The listing builds one solid part. Answer for the finished solid, in the listing's coordinates (mm). Face numbers are marked on the shaded views. A direction names the side the tool comes from. Coordinates: 2 decimals unless noted, no trailing zeros. Write each loop counter-clockwise with the first axis right and the second up, starting at its lowest first coordinate (ties: lowest second). Pieces come first, ordered by that corner, then holes.
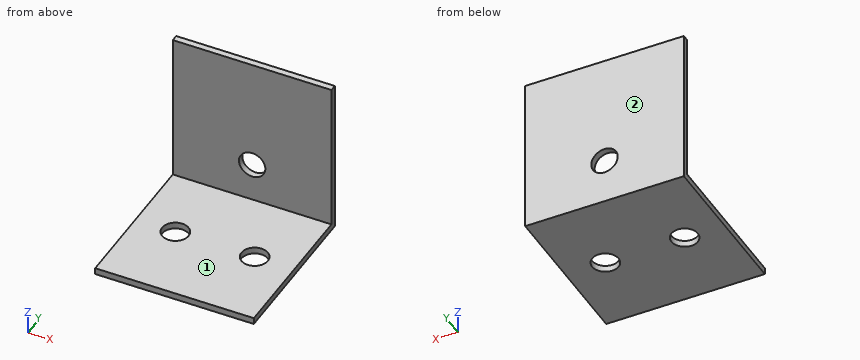
from build123d import *

# Parameters (mm, degrees)
F1_DEPTH = 38.1
F3_D     = 6.35
F5_D     = 6.35


with BuildPart() as f1:
    # F0 (on Right) → F1 (new body)
    with BuildSketch(Plane.YZ):
        Polygon((0, 1.5875), (0, 0), (38.1, 0), (38.1, 1.5875), (38.1, 38.1), (36.5125, 38.1), (36.5125, 1.5875), align=None)
    extrude(amount=F1_DEPTH)

    # F3 (through all)
    with Locations(Plane.XZ.offset(-36.5125)):
        with Locations((19.05, 11)):
            Hole(F3_D / 2)

    # F5 (through all)
    with Locations(Plane(origin=(0, 0, 0), x_dir=(1, 0, 0), z_dir=(0, 0, -1))):
        with Locations((9.525, -19.05), (28.575, -19.05)):
            Hole(F5_D / 2)


solid = f1.part
1. A tool of negligible diameter and unlimited length cuts with its end or side. For the marked faces 1 and 2, from which of +Z, -Z, +X, -X, +Y, -Y can it reach the whole face along a straight path? Write none if from no direction.
Results found:
face 1: +Z, +X, -X, -Y
face 2: +Z, -Z, +X, -X, +Y
2. Section A-A on x = 19.05 is taken. Give the vertices of the cut face in (y, z) (1 decimal).
Results found:
outline: (0, 0) - (38.1, 0) - (38.1, 7.8) - (36.5, 7.8) - (36.5, 1.6) - (0, 1.6) - close; (36.5, 14.2) - (38.1, 14.2) - (38.1, 38.1) - (36.5, 38.1) - close
3. Section D-D on x = 23.5 is taken. Give the vertices of the cut face in (y, z).
Results found:
outline: (0, 0) - (38.1, 0) - (38.1, 38.1) - (36.51, 38.1) - (36.51, 1.59) - (0, 1.59) - close
4. Find the intervals of material crossed by L1, parallel to X at y = 19.05, z = 0.7; L2, parallel to Y at x = 3.5, z = 10.5; L3, parallel to Z at x = 19, y = 6, in increasing order.
Results found:
L1: x = 0 to 6.35, 12.7 to 25.4, 31.75 to 38.1
L2: y = 36.51 to 38.1
L3: z = 0 to 1.59
5. Flat-ended cylindrical pins translate along their axes: P1, Ø7.5, axis at x = 9.525, y = 19.05, coming from the +Z side; P2, Ø10, axis at x = 15.5, z = 28.5, coming from the -Y side; P3, Ø6, axis at y = 32, z = 30, coming from the +X side. Find the tip coordinate at first contact, or state that the pin passes through.
Results found:
P1: stops at z = 1.59
P2: stops at y = 36.51
P3: passes through
6. Section C-C on z = 11 is taken. Give the vertices of the cut face in (x, y) (1 decimal), then the cut area to 3 significant figures.
Results found:
outline: (0, 36.5) - (15.9, 36.5) - (15.9, 38.1) - (0, 38.1) - close; (22.2, 36.5) - (38.1, 36.5) - (38.1, 38.1) - (22.2, 38.1) - close
area: 50.4 mm2
7. Section B-B on y = 19.05 is taken. Give the vertices of the cut face in (x, z).
Results found:
outline: (0, 0) - (6.35, 0) - (6.35, 1.59) - (0, 1.59) - close; (12.7, 0) - (25.4, 0) - (25.4, 1.59) - (12.7, 1.59) - close; (31.75, 0) - (38.1, 0) - (38.1, 1.59) - (31.75, 1.59) - close
